Design review of the part shown in the three views and the two pictorial views. Dimensions are in mm from the part's minimum x, y and z. Round coordinates to 2 decimals unless told otherwise and drop trailing zeros. Loops run counter-clockwise (first coordinate to the right, second up) from the corner with the lowest first, then second, coordinate; pieces in that order, holes last. Notation, with made-up numbers: (5.25, 50.5) - (25.25, 50.5) arc R21 cw to (25.25, 62.5) - close; hole circle Ø11 at (33, -28.5). An arc over 180 degrees is marked (long way). Return JSON: item names as keys, results as strings. Group by question number.
(1) We need section D-D, the plane x = 10.5. Write out the cut boundary in (y, z) (3 decimals).
(2) We need section A-A, the plane z = 10. Write out the cut boundary in (x, y) (3 decimals).
(3) Wall thickness on L1, parallel to X at y = 1.3, z = 60 (3 decimals); L2, parallel to X at y = 0.6, z = 62.5; L3, parallel to X at y = 2.5, z = 31: over which ranges is each line inside the solid? List them lowest first. Write a range as [from, to].
(4) We need section B-B, the plane y = 0.6. Write out the cut boundary in (x, z) (3 decimals).
(5) We need section C-C, the plane x = 139.5. Write out the cut boundary in (y, z) (3 decimals), and give its area (3 significant figures).
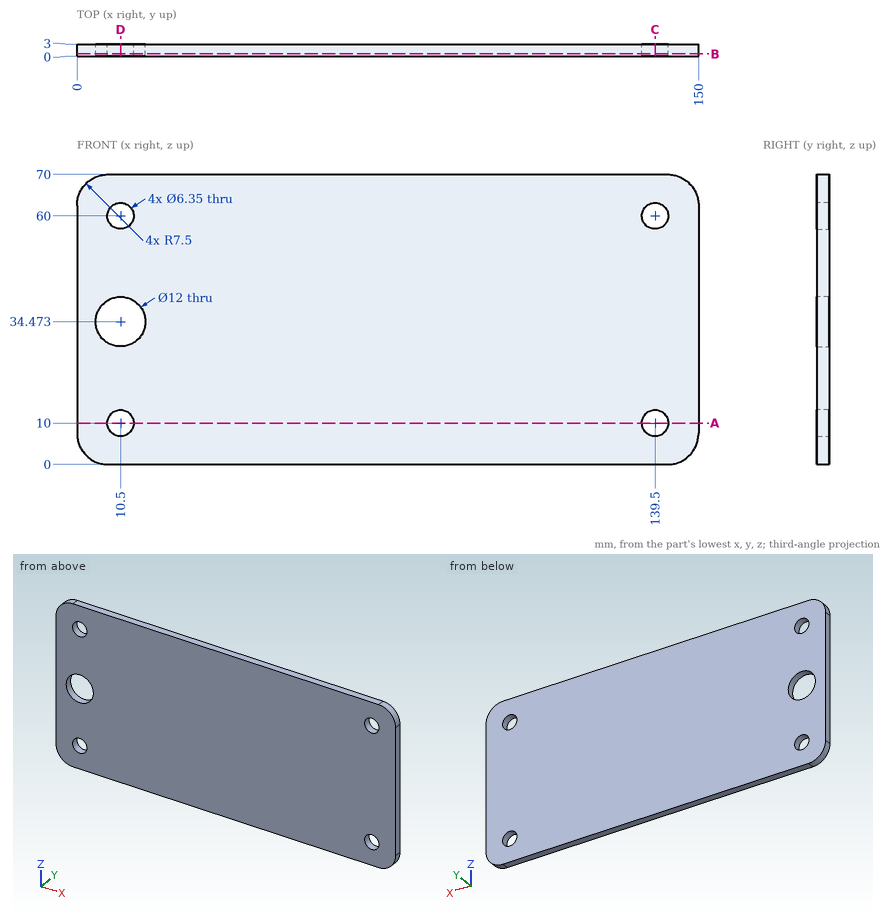
Solutions:
{
 "1": {"outline": "(0, 0) - (3, 0) - (3, 6.825) - (0, 6.825) - close; (0, 13.175) - (3, 13.175) - (3, 28.473) - (0, 28.473) - close; (0, 40.473) - (3, 40.473) - (3, 56.825) - (0, 56.825) - close; (0, 63.175) - (3, 63.175) - (3, 70) - (0, 70) - close"},
 "2": {"outline": "(0, 0) - (7.325, 0) - (7.325, 3) - (0, 3) - close; (13.675, 0) - (136.325, 0) - (136.325, 3) - (13.675, 3) - close; (142.675, 0) - (150, 0) - (150, 3) - (142.675, 3) - close"},
 "3": {"L1": "[0, 7.325], [13.675, 136.325], [142.675, 150]", "L2": "[0, 8.54], [12.46, 137.54], [141.46, 150]", "L3": "[0, 5.61], [15.39, 150]"},
 "4": {"outline": "(0, 7.5) arc R7.5 ccw to (7.5, 0) - (142.5, 0) arc R7.5 ccw to (150, 7.5) - (150, 62.5) arc R7.5 ccw to (142.5, 70) - (7.5, 70) arc R7.5 ccw to (0, 62.5) - close; hole circle Ø12 at (10.5, 34.473); hole circle Ø6.35 at (10.5, 10); hole circle Ø6.35 at (10.5, 60); hole circle Ø6.35 at (139.5, 10); hole circle Ø6.35 at (139.5, 60)"},
 "5": {"outline": "(0, 0) - (3, 0) - (3, 6.825) - (0, 6.825) - close; (0, 13.175) - (3, 13.175) - (3, 56.825) - (0, 56.825) - close; (0, 63.175) - (3, 63.175) - (3, 70) - (0, 70) - close", "area": "172 mm^2"}
}
